Geometry check sheet. Reference: drawing and pictorial views, mm from the part's lowest x, y, z. Coordinates: 2 decimals unless noted, no trailing zeros. Write each loop counter-clockwise with the first axis right and the second up, starting at its lowest first coordinate (ties: lowest second). Pieces come first, ordered by that corner, then holes. Notation, with made-up numbers: (74, 72) -> (127, 72) arc R16 cw to (127, 97) -> close; hole circle Ø2 at (-22.75, 57.5). An arc over 180 degrees is marked (long way). Use a Markdown table: item, result. Add a question column.
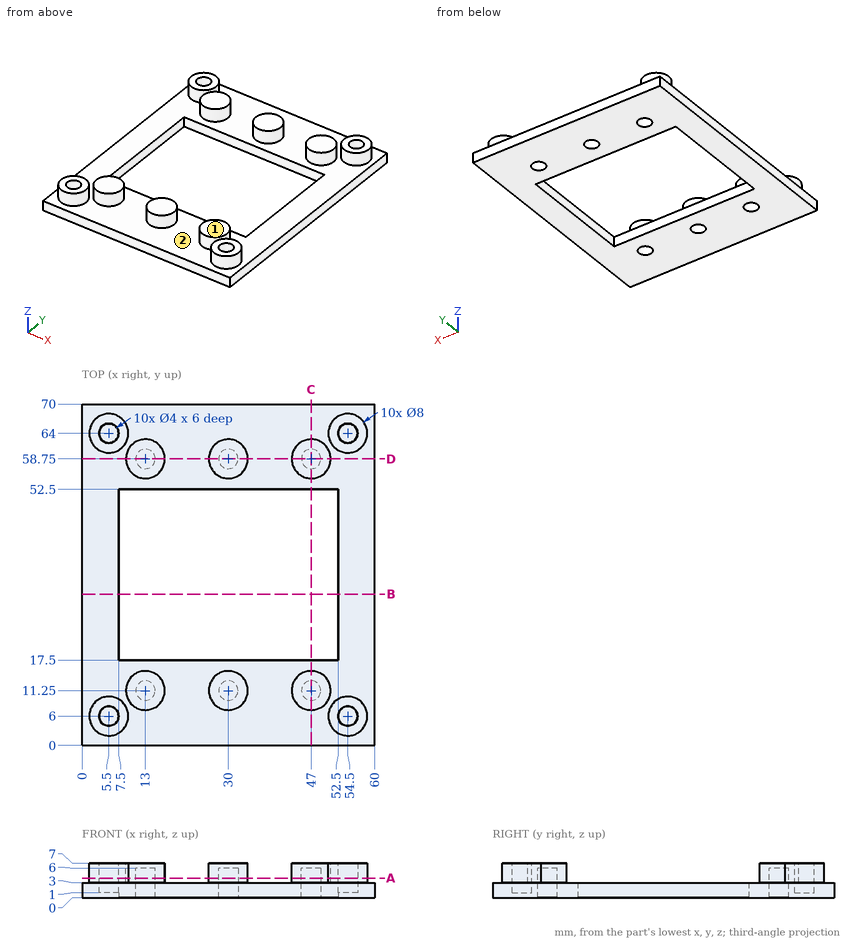
1) Cross-section at A-A on z = 4. Give the number of separate pieces and of enclosed holes in the cut face, then the cut area to 3 significant figures.
2) Gauge pin test, flat ends, axial feed: pin 1 (6.5 mm diameter, centred on x = 54.5, y = 64, fed in from +Z); pin 2 (1.2 mm diameter, centred on x = 47.5, y = 11.5, fed in from -Z); pin 3 (1.5 mm diameter, centred on x = 13.5, z = 5, fed in from -Y). Record the tip position at first contact, or that the pin passes through.
3) Cross-section at B-B on y = 31. Record the boundary of the cut face in (x, z).
4) Cross-section at D-D on y = 58.75. Record the boundary of the cut face in (x, z), then the cut area to 3 significant figures.
5) Cross-section at C-C on x = 47. Record the boundary of the cut face in (y, z), then the cut area to 3 significant figures.
6) Thickness scan on L1, parallel to Y at x = 54.5, z = 2.3; L2, parallel to Y at x = 30, z = 3.7; L3, parallel to Y at x = 5.5, z = 5.55. Record the ranges inside material, lowest first.
7) Release check for a two-part mould opening along Y. For the marked faces 1 and 2 record: released by +Y, released by -Y, zero draft, split by the parting line, or undercut.
Returned:
| question | item | result |
|---|---|---|
| 1 | separate pieces | 10 |
| 1 | enclosed holes | 10 |
| 1 | area | 377 mm² |
| 2 | pin 1 | stops at z = 7 |
| 2 | pin 2 | stops at z = 6 |
| 2 | pin 3 | stops at y = 7.25 |
| 3 | outline | (0, 0) -> (7.5, 0) -> (7.5, 3) -> (0, 3) -> close; (52.5, 0) -> (60, 0) -> (60, 3) -> (52.5, 3) -> close |
| 4 | outline | (0, 0) -> (11, 0) -> (11, 6) -> (15, 6) -> (15, 0) -> (28, 0) -> (28, 6) -> (32, 6) -> (32, 0) -> (45, 0) -> (45, 6) -> (49, 6) -> (49, 0) -> (60, 0) -> (60, 3) -> (51, 3) -> (51, 7) -> (43, 7) -> (43, 3) -> (34, 3) -> (34, 7) -> (26, 7) -> (26, 3) -> (17, 3) -> (17, 7) -> (9, 7) -> (9, 3) -> (0, 3) -> close |
| 4 | area | 204 mm² |
| 5 | outline | (0, 0) -> (9.25, 0) -> (9.25, 6) -> (13.25, 6) -> (13.25, 0) -> (17.5, 0) -> (17.5, 3) -> (15.25, 3) -> (15.25, 7) -> (7.25, 7) -> (7.25, 3) -> (0, 3) -> close; (52.5, 0) -> (56.75, 0) -> (56.75, 6) -> (60.75, 6) -> (60.75, 0) -> (70, 0) -> (70, 3) -> (62.75, 3) -> (62.75, 7) -> (54.75, 7) -> (54.75, 3) -> (52.5, 3) -> close |
| 5 | area | 121 mm² |
| 6 | L1 | y = 0 to 4, 8 to 62, 66 to 70 |
| 6 | L2 | y = 7.25 to 9.25, 13.25 to 15.25, 54.75 to 56.75, 60.75 to 62.75 |
| 6 | L3 | y = 2 to 4, 8 to 10, 60 to 62, 66 to 68 |
| 7 | face 1 | zero draft |
| 7 | face 2 | undercut |
